Could you check a few things on this model? Use its own coordinates, in mm. A direction names the side the tool comes from. Coordinates: 2 decimals unless noted, no trailing zeros. Write each loop counter-clockwise with the first axis right and the second up, starting at its lowest first coordinate (ties: lowest second). Pieces come first, ordered by that corner, then holes. Notation, with made-up numbers: M 24.5,-11.75 L 52.5,-11.75 A25 ccw 52.5,2.25 Z; hole C 66.25,68 d1. An arc over 180 degrees is marked long. Answer as CSV lines item,"result". Start each with the question number.
Item 1: Suppose I cut it at A-A, the plane z = 16. Write out the boundary of the cut face in (x, y).
Item 2: I'm going to push flat-ended pins straight in: P1, Ø8, axis at x = 2, z = 42.5, coming from the -Y side; P2, Ø5, axis at x = -5, z = 35.5, coming from the -Y side; P3, Ø8, axis at x = 3, z = 15.5, coming from the +Y side. Where does each tip first touch, or does it pass through?
Item 3: On a 3-axis mill with a long thin cutter (end or side, diameter ignored), from which of +Z, -Z, +X, -X, +Y, -Y can I reach the whole of each face in a straight line? I mean faces 1 (the cylindrical face through (-7.137, 0.314, 28.72)), 2 (the flat face through (8.62, -5.07, 4.44)). Say none if no direction works.
Item 4: If I drill on line 1 along Z through (x, y) = (9, -1); line 2 along Y through (x, z) = (0, 26); line 3 along X through (y, z) = (1.5, 14), over which ranges is the centre line in solid material (lowest first)? Write a range as [from, to].
```python
from build123d import *

# Parameters (mm, degrees)
SALIENTE_EXTRUIR1_DEPTH = 9
CROQUIS2_R              = 7.14375
SALIENTE_EXTRUIR2_DEPTH = 40
CROQUIS3_R              = 25.754458297
CROQUIS3_R_2            = 10
CORTAR_EXTRUIR1_DEPTH   = 3
CORTAR_EXTRUIR1_DRAFT   = -63


with BuildPart() as part:
    # Croquis1 → Saliente-Extruir1 (new body)
    with BuildSketch(Plane.XY):
        Polygon((11.547005384, 0), (5.773502692, 10), (-5.773502692, 10), (-11.547005384, 0), (-5.773502692, -10), (5.773502692, -10), align=None)
    extrude(amount=SALIENTE_EXTRUIR1_DEPTH)

    # Croquis2 → Saliente-Extruir2 (add)
    with BuildSketch(Plane.XY.offset(9)):
        Circle(CROQUIS2_R)
    extrude(amount=SALIENTE_EXTRUIR2_DEPTH)


with BuildPart() as cortar_extruir1_tool:
    # Croquis3 → Cortar-Extruir1 (with draft: the straight prism first)
    with BuildSketch(Plane(origin=(0, 0, 0), x_dir=(-1, 0, 0), z_dir=(0, 0, -1))):
        Circle(CROQUIS3_R)
        Circle(CROQUIS3_R_2, mode=Mode.SUBTRACT)
    extrude(amount=-CORTAR_EXTRUIR1_DEPTH)
    # Cortar-Extruir1: the draft: its side faces are tilted about the plane it starts from
    cortar_extruir1_sides = [cortar_extruir1_tool.faces().sort_by_distance(p)[0] for p in [
        (25.754458297, 0, 1.5),
        (10, 0, 1.5),
    ]]
    draft(cortar_extruir1_sides, Plane(origin=(0, 0, 0), x_dir=(-1, 0, 0), z_dir=(0, 0, -1)), CORTAR_EXTRUIR1_DRAFT)


with BuildPart() as part_1:
    add(part.part)

    # Cortar-Extruir1: cut by cortar_extruir1_tool
    add(cortar_extruir1_tool.part, mode=Mode.SUBTRACT)


solid = part_1.part
```
Ans:
1,outline,"C 0,0 d14.29"
2,P1,"stops at y = -7.14"
2,P2,"stops at y = -6.69"
2,P3,"stops at y = 7.14"
3,face 1,"+Z"
3,face 2,"+Z, -Z, +X, -Y"
4,line 1,"z = [0, 9]"
4,line 2,"y = [-7.14, 7.14]"
4,line 3,"x = [-6.98, 6.98]"
